The model under review builds one solid part; all positions refer to its coordinate system, in mm. Coordinates: 2 decimals unless noted, no trailing zeros. Loops run counter-clockwise (first coordinate to the right, second up) from the corner with the lowest first, then second, coordinate; pieces in that order, holes last. Notation, with made-up numbers: M 47,-12 L 60,-12 A13 cw 60,6 Z; hole C 47,89 d10. An arc over 180 degrees is marked long. One line per item, written item: value.
```python
from build123d import *

# Parameters (mm, degrees)
SKETCH1_R           = 2
SKETCH1_R_2         = 2.5
BOSS_EXTRUDE1_DEPTH = 4
CUT_EXTRUDE2_DEPTH  = 23
CHAMFER2_SIZE       = 1


with BuildPart() as part:
    # Sketch1 → Boss-Extrude1 (new body)
    with BuildSketch(Plane(origin=(0, 0, 0), x_dir=(1, 0, 0), z_dir=(0, 1, 0))):
        with BuildLine():
            Line((25.625, 28.625), (-25.625, 28.625))
            ThreePointArc((-25.625, 28.625), (-27.746320344, 27.746320344), (-28.625, 25.625))
            Line((-28.625, 25.625), (-28.625, -25.625))
            ThreePointArc((-28.625, -25.625), (-27.746320344, -27.746320344), (-25.625, -28.625))
            Line((-25.625, -28.625), (25.625, -28.625))
            ThreePointArc((25.625, -28.625), (27.746320344, -27.746320344), (28.625, -25.625))
            Line((28.625, -25.625), (28.625, 25.625))
            ThreePointArc((28.625, 25.625), (27.746320344, 27.746320344), (25.625, 28.625))
        make_face()
        with Locations(Location((-15.5, 15.5, 0), (0, 0, 270))):
            Circle(SKETCH1_R, mode=Mode.SUBTRACT)
        with Locations(Location((-23.57, 23.57, 0), (0, 0, 270))):
            Circle(SKETCH1_R_2, mode=Mode.SUBTRACT)
        with Locations(Location((23.57, 23.57, 0), (0, 0, 270))):
            Circle(SKETCH1_R_2, mode=Mode.SUBTRACT)
        with Locations(Location((15.5, 15.5, 0), (0, 0, 270))):
            Circle(SKETCH1_R, mode=Mode.SUBTRACT)
        with Locations(Location((15.5, -15.5, 0), (0, 0, 270))):
            Circle(SKETCH1_R, mode=Mode.SUBTRACT)
        with Locations(Location((-15.5, -15.5, 0), (0, 0, 270))):
            Circle(SKETCH1_R, mode=Mode.SUBTRACT)
        with Locations(Location((-23.57, -23.57, 0), (0, 0, 270))):
            Circle(SKETCH1_R_2, mode=Mode.SUBTRACT)
        with Locations(Location((23.57, -23.57, 0), (0, 0, 270))):
            Circle(SKETCH1_R_2, mode=Mode.SUBTRACT)
    extrude(amount=BOSS_EXTRUDE1_DEPTH)

    # Sketch3 → Cut-Extrude2 (cut)
    with BuildSketch(Plane.XY.offset(11.5)):
        Polygon((-28.125, 4), (-27.125, 3), (-26.125, 4), align=None)
        Polygon((-25.125, 4), (-24.125, 3), (-23.125, 4), align=None)
        Polygon((-22.125, 4), (-21.125, 3), (-20.125, 4), align=None)
        Polygon((-19.125, 4), (-18.125, 3), (-17.125, 4), align=None)
        Polygon((-16.125, 4), (-15.125, 3), (-14.125, 4), align=None)
        Polygon((-13.125, 4), (-12.125, 3), (-11.125, 4), align=None)
        Polygon((-10.125, 4), (-9.125, 3), (-8.125, 4), align=None)
        Polygon((-7.125, 4), (-6.125, 3), (-5.125, 4), align=None)
        Polygon((-4.125, 4), (-3.125, 3), (-2.125, 4), align=None)
        Polygon((-1.125, 4), (-0.125, 3), (0.875, 4), align=None)
        Polygon((1.875, 4), (2.875, 3), (3.875, 4), align=None)
        Polygon((4.875, 4), (5.875, 3), (6.875, 4), align=None)
        Polygon((7.875, 4), (8.875, 3), (9.875, 4), align=None)
        Polygon((10.875, 4), (11.875, 3), (12.875, 4), align=None)
        Polygon((13.875, 4), (14.875, 3), (15.875, 4), align=None)
        Polygon((16.875, 4), (17.875, 3), (18.875, 4), align=None)
        Polygon((19.875, 4), (20.875, 3), (21.875, 4), align=None)
        Polygon((22.875, 4), (23.875, 3), (24.875, 4), align=None)
        Polygon((25.875, 4), (26.875, 3), (27.875, 4), align=None)
    extrude(amount=-CUT_EXTRUDE2_DEPTH, mode=Mode.SUBTRACT)

    # Chamfer2
    chamfer2_edges = [part.edges().sort_by_distance(p)[0] for p in [
        (26.875, 4, -11.5),
        (23.875, 4, -11.5),
        (20.875, 4, -11.5),
        (17.875, 4, -11.5),
        (14.875, 4, -11.5),
        (11.875, 4, -11.5),
        (8.875, 4, -11.5),
        (5.875, 4, -11.5),
        (2.875, 4, -11.5),
        (-0.125, 4, -11.5),
        (-3.125, 4, -11.5),
        (-6.125, 4, -11.5),
        (-9.125, 4, -11.5),
        (-12.125, 4, -11.5),
        (-15.125, 4, -11.5),
        (-18.125, 4, -11.5),
        (-21.125, 4, -11.5),
        (-24.125, 4, -11.5),
        (-27.125, 4, -11.5),
        (26.875, 4, 11.5),
        (23.875, 4, 11.5),
        (20.875, 4, 11.5),
        (17.875, 4, 11.5),
        (14.875, 4, 11.5),
        (11.875, 4, 11.5),
        (8.875, 4, 11.5),
        (5.875, 4, 11.5),
        (2.875, 4, 11.5),
        (-0.125, 4, 11.5),
        (-3.125, 4, 11.5),
        (-6.125, 4, 11.5),
        (-9.125, 4, 11.5),
        (-12.125, 4, 11.5),
        (-15.125, 4, 11.5),
        (-18.125, 4, 11.5),
        (-21.125, 4, 11.5),
        (-24.125, 4, 11.5),
        (-27.125, 4, 11.5),
    ]]
    chamfer(chamfer2_edges, length=CHAMFER2_SIZE - 0.0001)  # a hair under: the kernel refuses the full size


solid = part.part
```
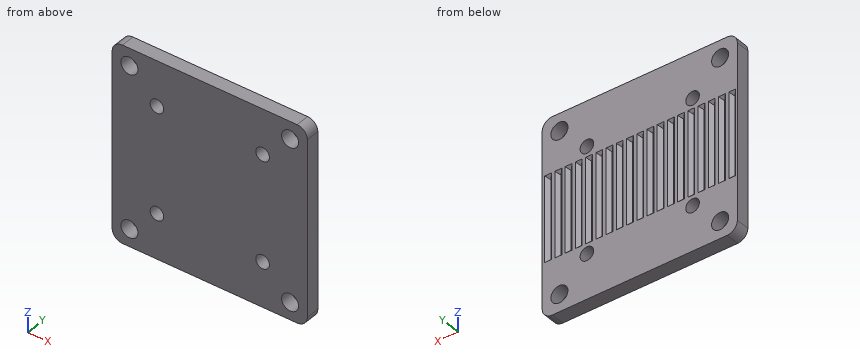
(1) To check wall thickness, follow L1, parallel to X at y = 3.1, z = -15.5 (3 decimals); L2, parallel to X at y = 2.1, z = 23.57 (3 decimals); L3, parallel to Z at x = -22.5, y = 2.5 (3 decimals). State the ranges of each line that lie inside material, in increasing order. Write a range as [from, to].
Checks:
L1: [-28.625, -17.5], [-13.5, 13.5], [17.5, 28.625]
L2: [-28.625, -26.07], [-21.07, 21.07], [26.07, 28.625]
L3: [-28.625, -25.829], [-21.311, 21.311], [25.829, 28.625]
(2) Add section B-B on y = 1.25. State how many separate pieces and enclosed holes the cut face has, then the cut area to 3 significant figures.
Checks:
separate pieces: 1
enclosed holes: 8
area: 3,140 mm^2
(3) Add section A-A on z = 23.57. State the section outline as (x, y) points (3 decimals), then the cut area to 3 significant figures.
Checks:
outline: M -28.625,0 L -26.07,0 L -26.07,4 L -28.625,4 Z; M -21.07,0 L 21.07,0 L 21.07,4 L -21.07,4 Z; M 26.07,0 L 28.625,0 L 28.625,4 L 26.07,4 Z
area: 189 mm^2
